The listing builds one solid part. Answer for the finished solid, in the listing's coordinates (mm). A direction names the side the tool comes from. Give positions to 0.01 mm unless a question says otherwise; leave off trailing zeros. Write each loop counter-clockwise with the first axis right and the second up, starting at its lowest first coordinate (ties: lowest second). Pieces come first, ordered by that corner, then holes. Notation, with made-up numbers: (-11, -12) -> (-1, -12) arc R16 cw to (-1, 2) -> close; hole circle Ø4 at (54.5, 47). An arc over 180 degrees is marked (long way). Put each result on its own line as item: value. Start each with the question number.
1) Flat-ended cylindrical pins translate along their axes: pin 1 Ø10 at (x, z) = (58.5, 9.5) entering from -Y; pin 2 Ø1 at (x, y) = (42, -4) entering from +Z; pin 3 Ø1 at (y, z) = (-9.5, 3) entering from +X; pin 4 Ø3 at (x, y) = (84, 11) entering from +Z. Find the tip coordinate at first contact, or state that the pin passes through.
2) Find the intervals of material crossed by line 1 along X through (y, z) = (-0.5, -10.25); line 2 along Z through (x, y) = (36, 3.75); line 3 along Y through (x, z) = (68.5, 1.75), in increasing order. Write a range as from..to.
3) A cutting plane is placed at A-A (x = 33.5). Write down the section's boundary in (y, z).
4) For faces 1 (the cylindrical face through (50.23, -1.73, -7.81)), 2 (the flat face through (-10, 0, 0)), determine the directions among +Z, -Z, +X, -X, +Y, -Y from which every point of the face is accessible in a straight line to the end or side of a thin tool.
Autodesk Inventor part; units mm, degrees
ref_plane "Work Plane1" through (1.525, 0, 0) normal (0, 0, 1) x (1, 0, 0)
ref_plane "YZ Plane" through (0, 0, 0) normal (1, 0, 0) x (0, 1, 0)
ref_plane "XZ Plane" through (0, 0, 0) normal (0, 1, 0) x (-1, 0, 0)
sketch "Sketch1" plane through (0, 0, 0) normal (0, 0, 1) x (1, 0, 0)
  line L0 (0, 11.245) -> (0, 8)
  line L1 (62, 8) -> (100, 8)
  line L2 (100, 8) -> (100, 0)
  line L3 (100, 0) -> (-0.8001, 0)
  line L4 (-20.9601, 0) -> (120.16, 0)
  line L5 (-0.8001, 0) -> (-0.8001, 11.245)
  line L6 (-0.8001, 11.245) -> (0, 11.245)
  line L7 (62, 8) -> (61.0797, 8)
  line L8 (61.0797, 8) -> (0, 8)
  line L9 (0, -2.249) -> (0, 13.494)
  dimension "d0" = 100
  dimension "d1" = 38
  dimension "d2" = 16
  dimension "d9" = 0.8001
  dimension "d10" = 22.49
  dimension "d13" = 0.9203
  dimension "d14" = 16
revolve "Body" add sketch "Sketch1" angle 360 about axis through (100, 0, 0) along (-1, 0, 0)
sketch "Sketch2" plane through (-0.8001, 0, 0) normal (-1, 0, 0) x (0, 0, 1)
  line L0 (0, 13.8564) -> (12, 6.9282)
  line L1 (12, 6.9282) -> (12, -6.9282)
  line L2 (12, -6.9282) -> (0, -13.8564)
  line L3 (0, -13.8564) -> (-12, -6.9282)
  line L4 (-12, -6.9282) -> (-12, 6.9282)
  line L5 (-12, 6.9282) -> (0, 13.8564)
  point P0 (0, 0)
  point P1 (0, 0)
  dimension "d11" = 24
extrude "Head" add sketch "Sketch2" along normal blind 9.2
sketch "Sketch4" plane through (0, 0, 0) normal (0, 0, 1) x (1, 0, 0)
  line L0 (-10.0001, 12) -> (-10.0001, 13.8564)
  line L1 (-10.0001, 13.8564) -> (-8.9283, 13.8564)
  line L2 (-8.9283, 13.8564) -> (-10.0001, 12)
  line L3 (-11.8401, 0) -> (1.0399, 0)
  line L4 (-0.8001, 13.8564) -> (-10.0001, 13.8564)
  line L5 (-10.0001, 6.9282) -> (-10.0001, 13.8564)
  dimension "d5" = 30
  dimension "d19" = 24
revolve "Chamfer1" cut sketch "Sketch4" angle 360 about axis through (-10, 0, 0) along (1, 0, 0)
thread "Thread"
chamfer "Chamfer2" distance 0.9202 distance2 0.9203 1 edges at (100, -8, 0) measured on face at (100, -0.9456, 1.8959)
ref_plane "Work Plane1" through (1.525, 0, 0) normal (0, 0, 1) x (1, 0, 0)
equation "\"d0\" = NLG"
equation "\"d1\" = GEL"
equation "\"d2\" = GD"
equation "\"d10\" = SD2"
equation "\"d14\" = BDM"
equation "\"d11\" = SW"
equation "\"d3\" = KOH - SD"
equation "\"d5\" = ANG1"
equation "\"d19\" = SW0"
equation "\"d15\" = GEL"
equation "\"d6\" = -0.5 * SPD + 0.5 * GD"
equation "\"NLG\" = 100"
equation "\"GD\" = NND"
equation "\"BDM\" = NND"
equation "\"KOH\" = 10"
equation "\"GEL\" = 38"
equation "\"SW\" = 24"
equation "\"SW0\" = SW"
equation "\"SPD\" = NND - 1.2269 * PTC"
equation "\"SD2\" = 22.49"
equation "\"SD\" = 0.8"
equation "\"ANG1\" = 30deg"
equation "\"GAL\" = 0.61345 * PTC"
equation "\"GUL\" = 0.61345 * PTC"
equation "\"RR\" = 0.6"
equation "\"GD1\" = THREADDIA - 1.2269 * PTC"
equation "\"THREADDIA\" = 16"
equation "\"SDH\" = SD2"
equation "\"TOA\" = 30deg"
equation "\"PTC\" = 1.5"
equation "\"NND\" = 16"
equation "\"E0\" = 1.155 * SW"
properties part number "ISO 8765 - M16 x 1.5 x 100" material "Stainless Steel, 440C"
Reply:
1. pin 1: stops at y = -6.61
1. pin 2: stops at z = 7.19
1. pin 3: stops at x = 0
1. pin 4: passes through
2. line 1: x = -10..0
2. line 2: z = -7.07..7.07
2. line 3: y = -7.81..7.81
3. outline: circle Ø16 at (0, 0)
4. face 1: +X
4. face 2: +Z, -Z, -X, +Y, -Y
